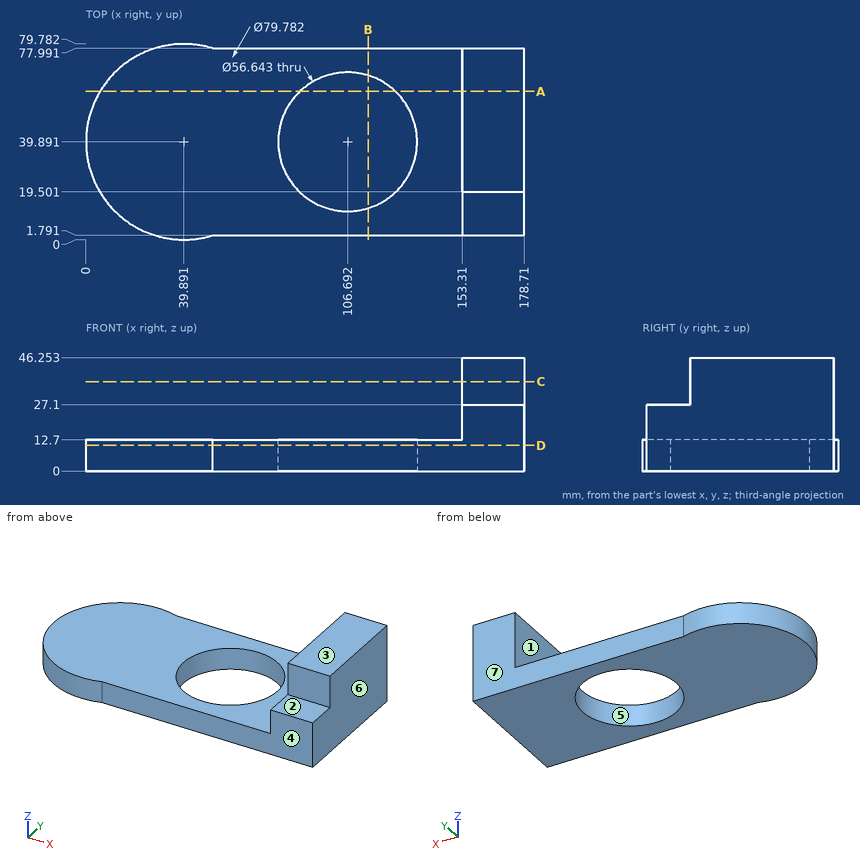
Study the drawing (mm; zero at the part's minimum x, y, z) and answer. A direction names the side the tool comes from. Give positions to 0.01 mm unless a question says otherwise; leave off trailing zeros. Write each loop counter-clockwise with the first axis right and the second up, starting at its lowest first coordinate (ties: lowest second). Pieces come first, ordered by that corner, then holes. Notation, with made-up numbers: M 63,-28.75 L 116,-28.75 A16 cw 116,-7.75 Z; hole C -29.5,73 d1. An arc over 180 degrees is marked long. Put each result on its own line as item: value. Start each with the question number.
1. The part is cut by section D-D, the plane z = 10.5. Give the vertices of the cut face in (x, y), and give its area (3 significant figures).
2. The part is cut by section A-A, the plane y = 60.5. Give the vertices of the cut face in (x, z), and give its area (3 significant figures).
3. For a pull along Y with two mould halves and no side action, classify the marked faces 4, 5, 6 and 7 as released by +Y, released by -Y, zero draft, split by the parting line, or undercut.
4. The part is cut by section C-C, the plane z = 36.5. Give the vertices of the cut face in (x, y), and give its area (3 significant figures).
5. Each of these flat-tipped pins is pushed along its axis until it touches: pin 1 Ø14 at (x, y) = (164, 7.5) entering from +Z; pin 2 Ø21.5 at (x, z) = (98, 7.5) entering from -Y; pin 3 Ø10 at (y, z) = (11, 11.5) entering from -X (1 decimal); pin 4 Ø8 at (x, z) = (147.5, 41.5) entering from +Y. Where does it stop, or does it pass through?
6. Which of the six approach directions +Z, -Z, +X, -X, +Y, -Y give full straight-line access (tool end or side, diameter ignored) to the marked faces 1, 2 and 3?
7. The part is cut by section B-B, the plane x = 115. Give the vertices of the cut face in (y, z) (1 decimal), and give its area (3 significant figures).
8. Consider line 1 along Y through (x, z) = (157, 40.5); line 2 along X through (y, z) = (35, 30.5); line 3 along Z through (x, y) = (62.5, 39). Determine where each line is inside the solid, lowest interval first.
Final values:
1. outline: M 51.71,1.79 L 178.71,1.79 L 178.71,77.99 L 51.71,77.99 A39.89 ccw long Z; hole C 106.69,39.89 d56.64
1. area: 10,600 mm²
2. outline: M 5.74,0 L 87.27,0 L 87.27,12.7 L 5.74,12.7 Z; M 126.12,0 L 178.71,0 L 178.71,46.25 L 153.31,46.25 L 153.31,12.7 L 126.12,12.7 Z
2. area: 2,560 mm²
3. face 4: released by -Y
3. face 5: undercut
3. face 6: zero draft
3. face 7: released by +Y
4. outline: M 153.31,19.5 L 178.71,19.5 L 178.71,77.99 L 153.31,77.99 Z
4. area: 1,490 mm²
5. pin 1: stops at z = 27.1
5. pin 2: stops at y = 1.79
5. pin 3: stops at x = 7.9
5. pin 4: passes through
6. face 1: +Z, -X, +Y, -Y
6. face 2: +Z, +X, -X, -Y
6. face 3: +Z, +X, -X, +Y, -Y
7. outline: M 1.8,0 L 12.8,0 L 12.8,12.7 L 1.8,12.7 Z; M 67,0 L 78,0 L 78,12.7 L 67,12.7 Z
7. area: 280 mm²
8. line 1: y = 19.5 to 77.99
8. line 2: x = 153.31 to 178.71
8. line 3: z = 0 to 12.7
